Autodesk Inventor part; units mm, degrees
ref_plane "YZ Plane" through (0, 0, 0) normal (1, 0, 0) x (0, 1, 0)
ref_plane "XZ Plane" through (0, 0, 0) normal (0, 1, 0) x (-1, 0, 0)
ref_plane "XY Plane" through (0, 0, 0) normal (0, 0, 1) x (1, 0, 0)
sketch "Sketch1" plane through (0, 0, 0) normal (0, 0, 1) x (1, 0, 0)
  line L0 (-7.5, 3) -> (7.5, 3)
  line L1 (7.5, 3) -> (7.5, -3)
  line L2 (7.5, -3) -> (-7.5, -3)
  line L3 (-7.5, -3) -> (-7.5, 3)
  circle A0 centre (0, 0) radius 4
  line L4 (-7.5, 3) -> (7.5, -3) construction
  dimension "d0" = 6
  dimension "d1" = 15
  dimension "d2" = 8
extrude "Extrusion1" add sketch "Sketch1" along normal blind 8 contours L0 A0 L2 L3 | L0 A0 L2 | L0 L1 L2 A0
extrude "Extrusion2" add sketch "Sketch1" against normal blind 8 contours A0 L0 | L0 A0 L2 | L2 A0
sketch "Sketch2" plane through (0, 0, 8) normal (0, 0, 1) x (1, 0, 0)
  circle A0 centre (0, 0) radius 1.5
  dimension "d7" = 3
extrude "Extrusion3" cut sketch "Sketch2" against normal through all
sketch "Sketch3" plane through (-7.5, 3, 8) normal (0, 1, 0) x (1, 0, 0)
  circle A0 centre (3.75, 4) radius 1.5
  circle A1 centre (11.25, 4) radius 1.5
  line L0 (3.75, 4) -> (0, 4)
  line L1 (0, 8) -> (0, 0)
  line L2 (3.75, 4) -> (7.5, 4)
  line L3 (7.5, 4) -> (11.25, 4)
  line L4 (11.25, 4) -> (15, 4)
  line L5 (15, 8) -> (15, 0)
  point P0 (7.5, 8)
  dimension "d10" = 3
  dimension "d11" = 3
extrude "Extrusion4" cut sketch "Sketch3" against normal through all
sketch "Sketch4" plane through (0, 0, -8) normal (0, 0, -1) x (-1, 0, 0)
  circle A0 centre (0, 0) radius 2.5
  line L0 (1.5, -2) -> (-1.5, -2)
  dimension "d14" = 5
  dimension "d15" = 4.5
extrude "Extrusion5" cut sketch "Sketch4" against normal blind 16.75 contours A0 L0 picked at (0.6276, -0.7851)
properties part number "wierd bearing interface part"
Input: part model. Units: mm. Frame: model coordinates. A direction names the side the tool comes from. Give positions to 0.01 mm unless a question says otherwise; leave off trailing zeros. Order: outer loops, then holes, each group sorted by start corner. A loop starts at its lowest first (then second) coordinate and runs counter-clockwise, first axis right, second up.
1. Section C-C on z = -2. Return the cut outline in (x, y).
Derived:
outline: circle Ø8 at (0, 0); hole (-1.5, -2) - (1.5, -2) arc R2.5 ccw (long way) to start
2. Mould query, pull axis X, two halves, no side actions, for faces 6 (the flat face through (0, -3.4, 0)), 7 (the flat face through (7.5, 0, 4)), 8 (the cylindrical face through (5.18, 0.04, 3.55)). Classes: released by +X, released by -X, zero draft, split by the parting line, or undercut.
Derived:
face 6: zero draft
face 7: released by +X
face 8: undercut
3. Section A-A on y = -1.75. Return the cut outline in (x, z).
Derived:
outline: (-7.5, 0) - (-3.6, 0) - (-3.6, -8) - (-1.79, -8) - (-1.79, 8) - (-7.5, 8) - close; (1.79, -8) - (3.6, -8) - (3.6, 0) - (7.5, 0) - (7.5, 8) - (1.79, 8) - close; hole circle Ø3 at (-3.75, 4); hole circle Ø3 at (3.75, 4)
4. Pin query (flat end, axial travel): pin 1 (4 mm diameter, centred on x = 2.5, z = 5, fed in from -Y); pin 2 (0.5 mm diameter, centred on x = 0.5, y = -3.5, fed in from +Z); pin 3 (1.5 mm diameter, centred on x = -5.5, y = -1, fed in from -Z). Return the tip coordinate at first contact, or that it passes through.
Derived:
pin 1: stops at y = -3
pin 2: stops at z = 0
pin 3: stops at z = 0
5. Reachability of faces 1 (the flat face through (0, 3, 4)), 2 (the flat face through (0, -2, 0)), 3 (the cylindrical face through (-0.867, -3.905, -3.944)), 4 (the flat face through (-2, 2, 8)), 5 (the flat face through (0, -3, 4)) from +Z, -Z, +X, -X, +Y, -Y: full face, straight path, thin tool, end or side. Return the list, or none.
Derived:
face 1: +Z, +X, -X, +Y
face 2: +Z, -Z
face 3: -Z
face 4: +Z, +X, -X, +Y, -Y
face 5: +Z, +X, -X, -Y
6. Section B-B on x = 0. Return the cut outline in (y, z), and give its area (3 significant figures).
Derived:
outline: (-4, -8) - (-2, -8) - (-2, 8) - (-3, 8) - (-3, 0) - (-4, 0) - close; (2.5, -8) - (4, -8) - (4, 0) - (3, 0) - (3, 8) - (2.5, 8) - close
area: 40.0 mm2
7. Material intervals for L1, parallel to X at y = -0.5, z = 4; L2, parallel to Z at x = -3.75, y = -0.25; L3, parallel to Y at x = 0, z = -1.25, sorted ascending.
Derived:
L1: x = -7.5 to -5.25, 5.25 to 7.5
L2: z = -8 to 2.5, 5.5 to 8
L3: y = -4 to -2, 2.5 to 4
8. Section D-D on y = 0.75. Return the cut outline in (x, z).
Derived:
outline: (-7.5, 0) - (-3.93, 0) - (-3.93, -8) - (-2.38, -8) - (-2.38, 3.38) arc R1.5 cw (long way) to (-2.38, 4.62) - (-2.38, 8) - (-7.5, 8) - close; (2.38, -8) - (3.93, -8) - (3.93, 0) - (7.5, 0) - (7.5, 8) - (2.38, 8) - (2.38, 4.62) arc R1.5 cw (long way) to (2.38, 3.38) - close
